Study the drawing (mm; zero at the part's minimum x, y, z) and answer. A direction names the side the tool comes from. Round coordinates to 2 decimals unless told otherwise and drop trailing zeros. Write each loop counter-clockwise with the first axis right and the second up, starting at its lowest first coordinate (ties: lowest second). Pieces come first, ordered by that corner, then holes.
(1) For the marked faces 1, 2 and 3, determine the directions among +Z, -Z, +X, -X, +Y, -Y from which every point of the face is accessible in a straight line to the end or side of a thin tool.
(2) A cutting plane is placed at B-B, the plane y = 46.5. Give the vertices of the cut face in (x, z), and give its area (3 significant figures).
(3) Each of these flat-tipped pins is pushed along its axis until it touches: pin 1 Ø2 at (y, z) = (45.5, 6) entering from -X; pin 2 Ø16.5 at (x, y) = (15, 41) entering from +Z; pin 3 Ø15.5 at (x, y) = (18.5, 6.5) entering from -Z. Where does it stop, or does it pass through?
(4) Find the intervals of material crossed by probe 1 along X at (y, z) = (36, 1.25); probe 2 along Y at (x, z) = (17.5, 12.25); probe 3 along Y at (x, z) = (17.5, 6), in increasing order.
(5) A cutting plane is placed at C-C, the plane y = 23. Give the vertices of the cut face in (x, z), and give its area (3 significant figures).
(6) The mould has two halves that part along Y. Classify the marked faces 4, 5, 6 and 7: +Y half, -Y half, draft (parallel to the pull), parting line (faces both ways), or undercut.
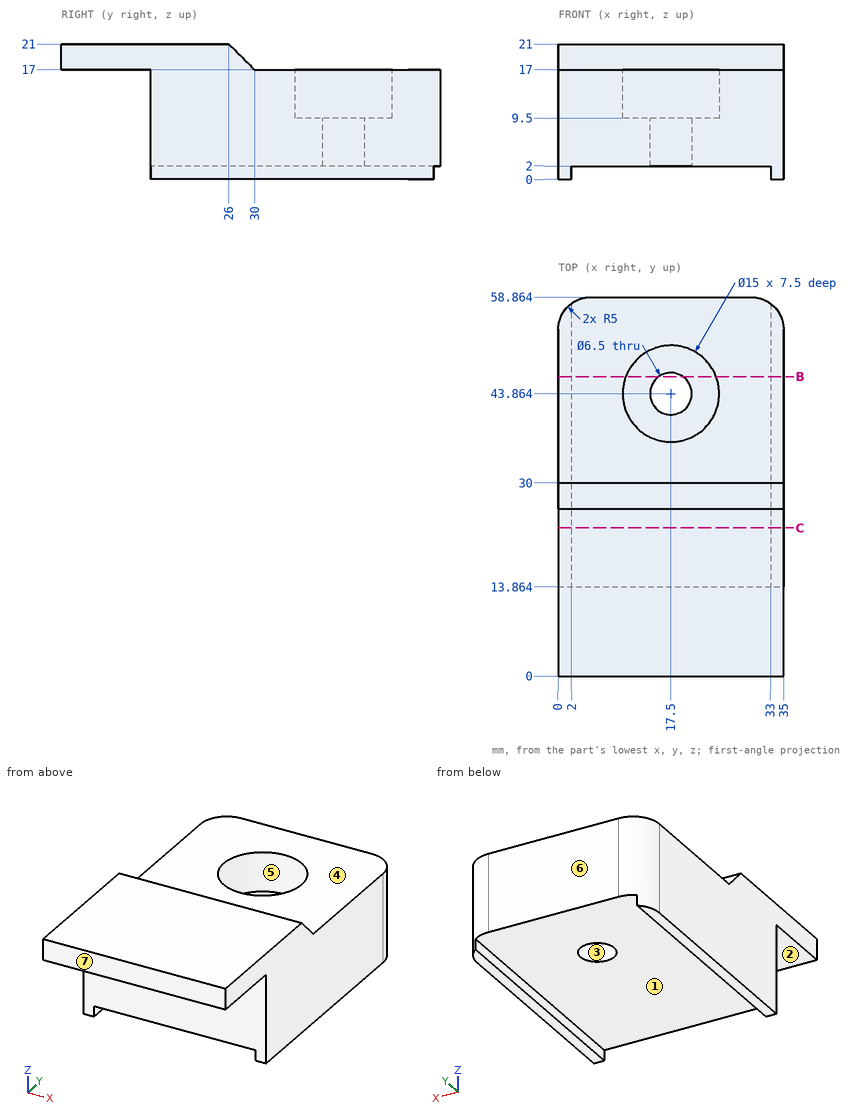
Solutions:
1. face 1: -Z, +Y, -Y
1. face 2: -Z, +X, -X, -Y
1. face 3: +Z, -Z
2. outline: (0, 0) - (2, 0) - (2, 2) - (15.6, 2) - (15.6, 9.5) - (10.48, 9.5) - (10.48, 17) - (0, 17) - close; (19.4, 2) - (33, 2) - (33, 0) - (35, 0) - (35, 17) - (24.52, 17) - (24.52, 9.5) - (19.4, 9.5) - close
2. area: 399 mm2
3. pin 1: stops at x = 0
3. pin 2: stops at z = 17
3. pin 3: stops at z = 2
4. probe 1: x = 0 to 2, 33 to 35
4. probe 2: y = 13.86 to 36.36, 51.36 to 58.86
4. probe 3: y = 13.86 to 40.61, 47.11 to 58.86
5. outline: (0, 0) - (2, 0) - (2, 2) - (33, 2) - (33, 0) - (35, 0) - (35, 21) - (0, 21) - close
5. area: 673 mm2
6. face 4: draft
6. face 5: undercut
6. face 6: +Y half
6. face 7: -Y half
